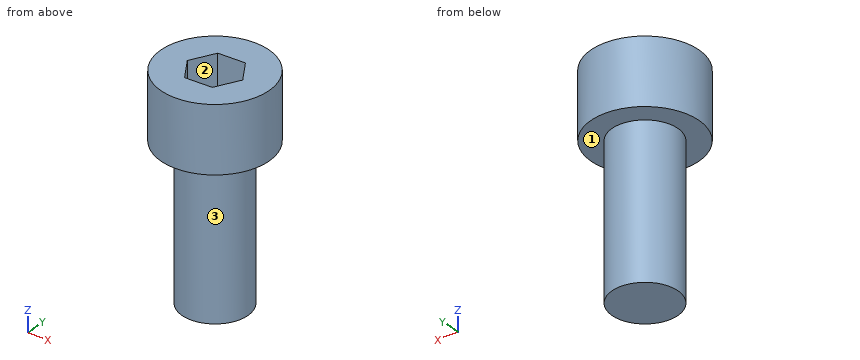
from build123d import *

# Parameters (mm, degrees)
SKETCH1_R           = 2.413
BOSS_EXTRUDE1_DEPTH = 11.1125
SKETCH2_R           = 3.9624
BOSS_EXTRUDE2_DEPTH = 4.826
CUT_EXTRUDE1_DEPTH  = 2.413


with BuildPart() as part:
    # Sketch1 → Boss-Extrude1 (new body)
    with BuildSketch(Plane.XY):
        Circle(SKETCH1_R)
    extrude(amount=BOSS_EXTRUDE1_DEPTH)

    # Sketch2 → Boss-Extrude2 (add)
    with BuildSketch(Plane.XY.offset(11.1125)):
        Circle(SKETCH2_R)
    extrude(amount=BOSS_EXTRUDE2_DEPTH)

    # Sketch3 → Cut-Extrude1 (cut)
    with BuildSketch(Plane.XY.offset(15.9385)):
        Polygon((0.940029384, 1.747595175), (-1.043447125, 1.687886915), (-1.98347651, -0.059708261), (-0.940029384, -1.747595175), (1.043447125, -1.687886915), (1.98347651, 0.059708261), align=None)
    extrude(amount=-CUT_EXTRUDE1_DEPTH, mode=Mode.SUBTRACT)


solid = part.part
Source: CAD feature listing. Evaluate the final solid. Frame: model axes, mm. Face numbers are marked on the shaded views. Round coordinates to 2 decimals unless told otherwise and drop trailing zeros. Write each loop counter-clockwise with the first axis right and the second up, starting at its lowest first coordinate (ties: lowest second). Pieces come first, ordered by that corner, then holes. Notation, with made-up numbers: (32, -22) - (43, -22) arc R19 ccw to (43, 2) - close; hole circle Ø7 at (4.25, 37). An arc over 180 degrees is marked (long way). Use CSV: the item, a comma, the result in double quotes. Start each with the question number.
(1) Cut plane B-B, the plane z = 12.5. Return loops of the section in (x, y), and give its area (3 significant figures).
(2) First-contact query: pin 1 Ø2 at (y, z) = (-0.5, 7.5) entering from -X. Flat tip, straight axial feed; report the tip coordinate or a pass-through.
(3) Cut plane C-C, the plane x = 0. Return loops of the section in (y, z), and give its area (3 significant figures).
(4) Cut plane D-D, the plane y = -2. Return loops of the section in (x, z), and give its area (3 significant figures).
(5) Material intervals for probe 1 along Z at (x, y) = (-1.75, -3); probe 2 along Z at (x, y) = (0.5, -1.5); probe 3 along X at (y, z) = (-1.5, 14.75), sorted ascending. Write a range as [from, to].
(6) Mould query, pull axis X, two halves, no side actions, for the marked faces 1, 2 and 3. Classes: pulls with the +X half, pulls with the -X half, needs draft (parallel to the pull), parting line crosses it, or undercut.
(7) Cut plane A-A, the plane y = -1. Return loops of the section in (x, z).
Geometry says:
1,outline,"circle Ø7.92 at (0, 0)"
1,area,"49.3 mm²"
2,pin 1,"x = -2.41"
3,outline,"(-3.96, 11.11) - (-2.41, 11.11) - (-2.41, 0) - (2.41, 0) - (2.41, 11.11) - (3.96, 11.11) - (3.96, 15.94) - (1.72, 15.94) - (1.72, 13.53) - (-1.72, 13.53) - (-1.72, 15.94) - (-3.96, 15.94) - close"
3,area,"83.6 mm²"
4,outline,"(-3.42, 11.11) - (-1.35, 11.11) - (-1.35, 0) - (1.35, 0) - (1.35, 11.11) - (3.42, 11.11) - (3.42, 15.94) - (-3.42, 15.94) - close"
4,area,"63.0 mm²"
5,probe 1,"[11.11, 15.94]"
5,probe 2,"[0, 13.53]"
5,probe 3,"[-3.67, -1.09], [1.14, 3.67]"
6,face 1,"needs draft"
6,face 2,"undercut"
6,face 3,"parting line crosses it"
7,outline,"(-3.83, 11.11) - (-2.2, 11.11) - (-2.2, 0) - (2.2, 0) - (2.2, 11.11) - (3.83, 11.11) - (3.83, 15.94) - (1.41, 15.94) - (1.41, 13.53) - (-1.4, 13.53) - (-1.4, 15.94) - (-3.83, 15.94) - close"
